The figure shows three views and two pictorial views of one solid part (mm, origin at its lowest corner). Answer the questions. A direction names the side the tool comes from. Give positions to 0.01 mm unless a question says otherwise; leave off trailing zeros. Loops run counter-clockwise (first coordinate to the right, second up) from the corner with the lowest first, then second, coordinate; pieces in that order, holes last. Notation, with made-up numbers: (-5, 10) - (37, 10) arc R25 cw to (37, 35) - close; hole circle Ø8 at (85, 13). An arc over 180 degrees is marked (long way). Use CSV: the item, a comma, the result in double quotes.
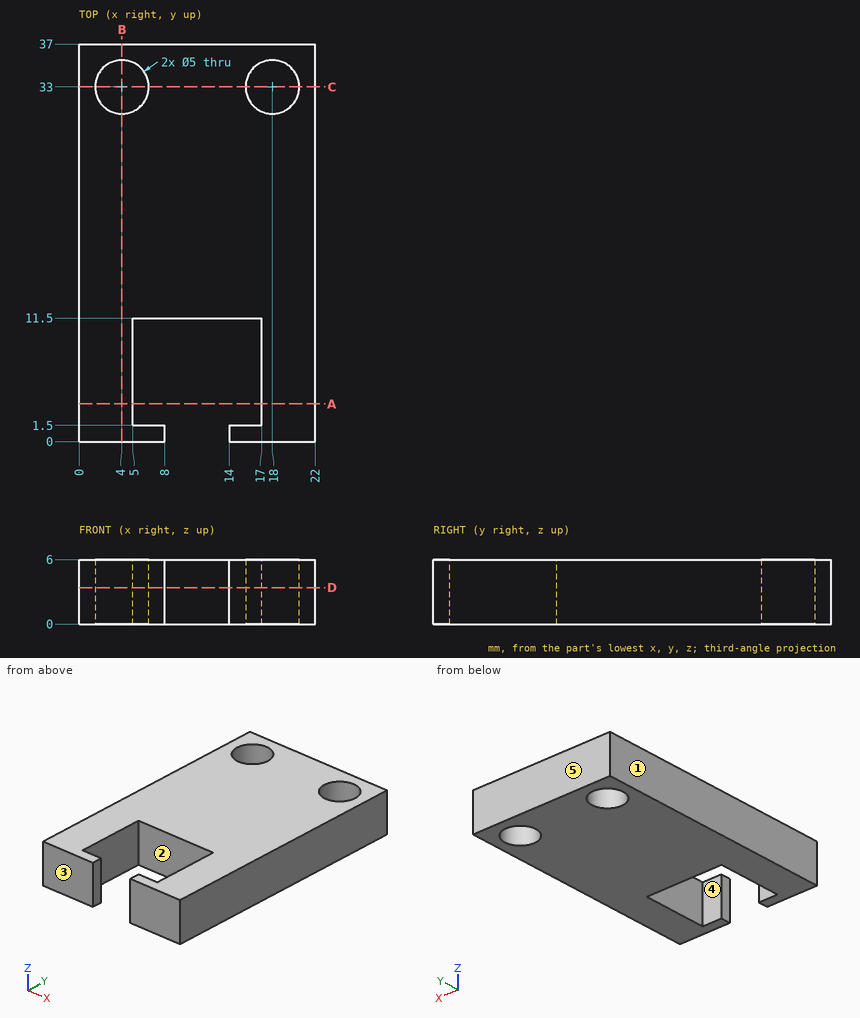
Item 1: A cutting plane is placed at B-B on x = 4. Determine the outline of the cut face in (y, z).
Determined:
outline,"(0, 0) - (30.5, 0) - (30.5, 6) - (0, 6) - close; (35.5, 0) - (37, 0) - (37, 6) - (35.5, 6) - close"
Item 2: For the marked faces 4 and 5, determine the directions among +Z, -Z, +X, -X, +Y, -Y from which every point of the face is accessible in a straight line to the end or side of a thin tool.
Determined:
face 4,"+Z, -Z"
face 5,"+Z, -Z, +X, -X, +Y"
Item 3: A cutting plane is placed at C-C on y = 33. Determine the outline of the cut face in (x, z).
Determined:
outline,"(0, 0) - (1.5, 0) - (1.5, 6) - (0, 6) - close; (6.5, 0) - (15.5, 0) - (15.5, 6) - (6.5, 6) - close; (20.5, 0) - (22, 0) - (22, 6) - (20.5, 6) - close"
Item 4: A cutting plane is placed at A-A on y = 3.5. Determine the outline of the cut face in (x, z), and give its area (3 significant figures).
Determined:
outline,"(0, 0) - (5, 0) - (5, 6) - (0, 6) - close; (17, 0) - (22, 0) - (22, 6) - (17, 6) - close"
area,"60.0 mm²"
Item 5: Given P1, Ø3, axis at y = 5, z = 2.5, coming from the -X side, flat-ended and moving along its own axis, determine where the tip first touches the part or whether it passes through.
Determined:
P1,"stops at x = 0"
Item 6: The mould has two halves that part along Y. Classify the marked faces 1, 2 and 3: pulls with the +Y half, pulls with the -Y half, needs draft (parallel to the pull), parting line crosses it, or undercut.
Determined:
face 1,"needs draft"
face 2,"undercut"
face 3,"pulls with the -Y half"
Item 7: A cutting plane is placed at D-D on z = 3.4. Determine the outline of the cut face in (x, y).
Determined:
outline,"(0, 0) - (8, 0) - (8, 1.5) - (5, 1.5) - (5, 11.5) - (17, 11.5) - (17, 1.5) - (14, 1.5) - (14, 0) - (22, 0) - (22, 37) - (0, 37) - close; hole circle Ø5 at (4, 33); hole circle Ø5 at (18, 33)"
Item 8: Find the intervals of material crossed by line 1 (Y direction, x = 18, z = 3.35); line 2 (Y direction, x = 14.5, z = 2.75); line 3 (X direction, y = 5, z = 4.2), in increasing order.
Determined:
line 1,"y = 0 to 30.5, 35.5 to 37"
line 2,"y = 0 to 1.5, 11.5 to 37"
line 3,"x = 0 to 5, 17 to 22"
